Geometry check sheet. Reference: drawing and pictorial views, mm from the part's lowest x, y, z. A direction names the side the tool comes from. Round coordinates to 2 decimals unless told otherwise and drop trailing zeros. Write each loop counter-clockwise with the first axis right and the second up, starting at its lowest first coordinate (ties: lowest second). Pieces come first, ordered by that corner, then holes. Notation, with made-up numbers: M 24,67.5 L 53,67.5 A8 ccw 53,76.5 Z; hole C 16.5,-1 d2. An arc over 180 degrees is marked long. Answer in a Markdown table with one row per item. Add a question column.
1. Go/stop test with flat-tipped pins: pin 1 Ø9.5 at (x, z) = (69.08, 25) entering from +Y; pin 2 Ø8 at (x, y) = (12, 10.5) entering from -Z; pin 3 Ø5 at (x, y) = (14, 10.5) entering from +Z. Record where each tip stops, or that it passes through.
2. Sectioned sample at D-D on y = 6.5. Record the cut outline in (x, z), plus the area to 3 significant figures.
3. Set-up check for the marked faces 1 and 2: record each of +Z, -Z, +X, -X, +Y, -Y from which the full face is reachable in a straight line by a thin tool's end or side.
4. Sectioned sample at C-C on z = 39. Record the cut outline in (x, y), plus the area to 3 significant figures.
5. Sectioned sample at A-A on z = 25. Record the cut outline in (x, y), plus the area to 3 significant figures.
6. Sectioned sample at B-B on x = 28. Record the cut outline in (y, z).
7. Material ranges on probe 1 along X at (y, z) = (1.1, 25); probe 2 along X at (y, z) = (9.5, 19); probe 3 along Y at (x, z) = (65, 3.5), recorded low to high.
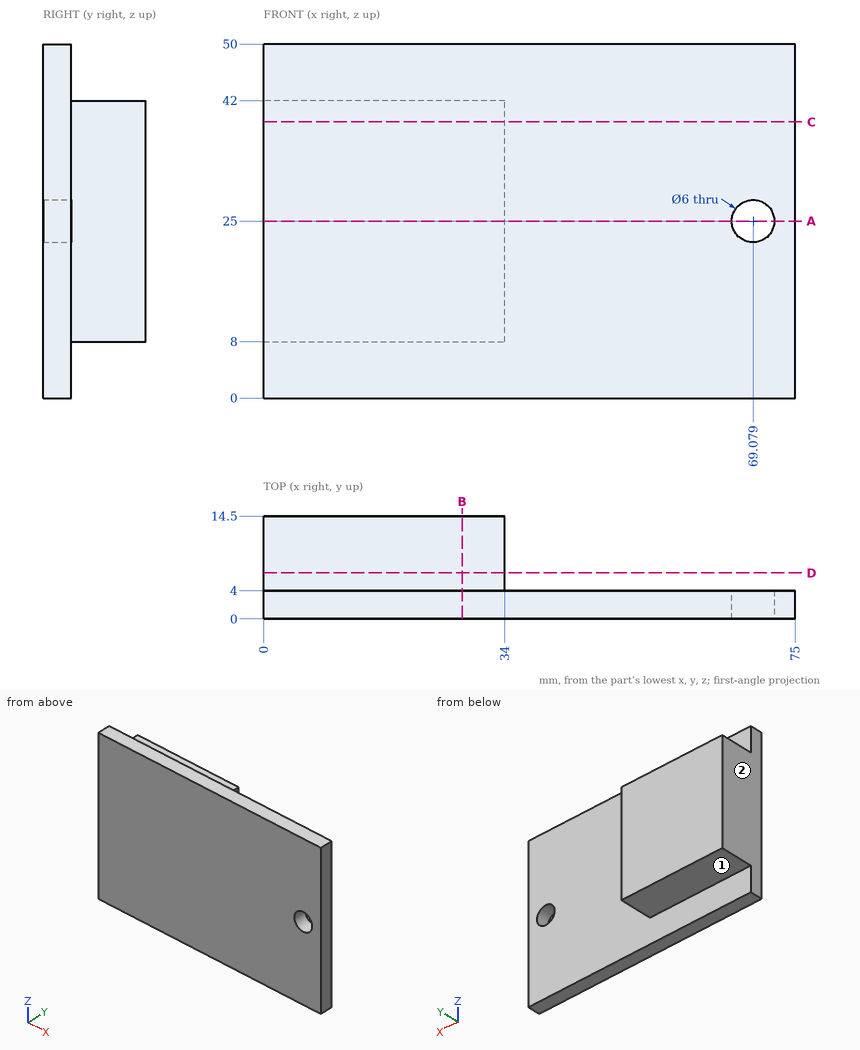
Geometry check:
| question | item | result |
|---|---|---|
| 1 | pin 1 | stops at y = 4 |
| 1 | pin 2 | stops at z = 8 |
| 1 | pin 3 | stops at z = 42 |
| 2 | outline | M 0,8 L 34,8 L 34,42 L 0,42 Z |
| 2 | area | 1,160 mm2 |
| 3 | face 1 | -Z, +X, -X, +Y |
| 3 | face 2 | +Z, -Z, -X, +Y, -Y |
| 4 | outline | M 0,0 L 75,0 L 75,4 L 34,4 L 34,14.5 L 0,14.5 Z |
| 4 | area | 657 mm2 |
| 5 | outline | M 0,0 L 66.08,0 L 66.08,4 L 34,4 L 34,14.5 L 0,14.5 Z; M 72.08,0 L 75,0 L 75,4 L 72.08,4 Z |
| 5 | area | 633 mm2 |
| 6 | outline | M 0,0 L 4,0 L 4,8 L 14.5,8 L 14.5,42 L 4,42 L 4,50 L 0,50 Z |
| 7 | probe 1 | x = 0 to 66.08, 72.08 to 75 |
| 7 | probe 2 | x = 0 to 34 |
| 7 | probe 3 | y = 0 to 4 |
